Here's how the part is built. I have some questions about the finished solid (model axes, mm). Round coordinates to 2 decimals unless told otherwise and drop trailing zeros. Loops run counter-clockwise (first coordinate to the right, second up) from the corner with the lowest first, then second, coordinate; pieces in that order, holes last. Notation, with made-up numbers: (-5, 52) - (11, 52) arc R28 cw to (11, 78) - close; hole circle Ø4 at (56.25, 67.5). An arc over 180 degrees is marked (long way). Answer as a JSON object with one key per item and string values. Group by question number.
1) I want a section at B-B, the plane x = 5.5. Please give me the cut outline in (y, z), then the cut area to 3 significant figures.
2) Will these pins go through, and if not, where does the flat tip stop? P1, Ø3, axis at x = 4.5, y = -1.5, coming from the +Z side; P2, Ø2, axis at x = 4.5, z = -4.5, coming from the -Y side.
3) I want a section at C-C, the plane y = -1.5. Please give me the cut outline in (x, z).
4) I want a section at A-A, the plane z = -0.95. Please give me the cut outline in (x, y).
5) If I drill on line 1 along Y through (x, z) = (-0.5, -1.65); line 2 along Y through (x, z) = (-6, -0.7); line 3 along X through (y, z) = (4, -3), over which ranges is the centre line in solid material (lowest first)? Write a range as [from, to].
from build123d import *

# Parameters (mm, degrees)
F0_R      = 7
F1_DEPTH  = 5
F2_R      = 7
F3_DEPTH  = 5
F1_FACE_R = 7
F4_DEPTH  = 5


with BuildPart() as f1:
    # F0 (on Top) → F1 (new body)
    with BuildSketch(Plane.XY):
        Circle(F0_R)
    extrude(amount=F1_DEPTH)

    # F2 (on Top) → F3 (join)
    with BuildSketch(Plane.XY):
        Circle(F2_R)
    extrude(amount=-F3_DEPTH)

    # F1_face (on face) → F4 (cut)
    with BuildSketch(Plane.XY.offset(5)):
        Circle(F1_FACE_R)
    extrude(amount=-F4_DEPTH, mode=Mode.SUBTRACT)


solid = f1.part
Outcome:
{
 "1": {"outline": "(-4.33, -5) - (4.33, -5) - (4.33, 0) - (-4.33, 0) - close", "area": "43.3 mm^2"},
 "2": {"P1": "z = 0", "P2": "y = -6.06"},
 "3": {"outline": "(-6.84, -5) - (6.84, -5) - (6.84, 0) - (-6.84, 0) - close"},
 "4": {"outline": "circle Ø14 at (0, 0)"},
 "5": {"line 1": "[-6.98, 6.98]", "line 2": "[-3.61, 3.61]", "line 3": "[-5.74, 5.74]"}
}
